Design review of the part built by this model. Coordinates are the model's own, in mm. Face numbers are marked on the shaded views. A direction names the side the tool comes from. Round coordinates to 2 decimals unless told otherwise and drop trailing zeros. Loops run counter-clockwise (first coordinate to the right, second up) from the corner with the lowest first, then second, coordinate; pieces in that order, holes last. Notation, with made-up numbers: M 42,44.5 L 79,44.5 A5 ccw 79,50.5 Z; hole C 49.5,46 d3. An arc over 180 degrees is marked long. Use a Markdown table: item, result.
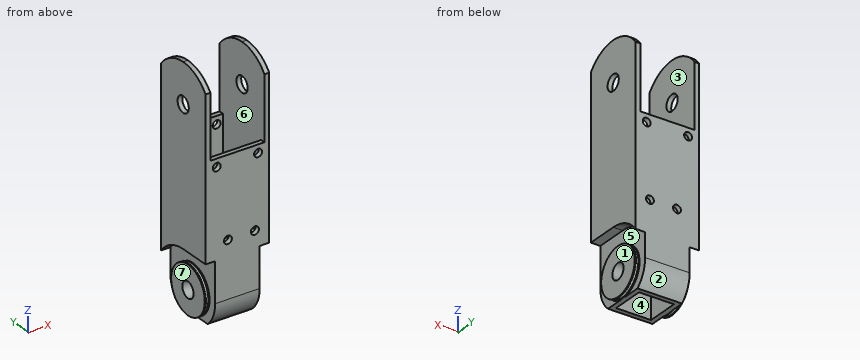
from build123d import *

# Parameters (mm, degrees)
CROQUIS1_W              = 40
CROQUIS1_H              = 40
SALIENTE_EXTRUIR1_DEPTH = 150
CROQUIS2_W              = 34
CROQUIS2_H              = 40
CORTAR_EXTRUIR1_DEPTH   = 50
CORTAR_EXTRUIR5_DEPTH   = 157.524758425
CROQUIS4_R              = 5
CORTAR_EXTRUIR6_DEPTH   = 157.524758425
CORTAR_EXTRUIR10_DEPTH  = 157.524758425
CROQUIS5_R              = 5
CORTAR_EXTRUIR7_DEPTH   = 157.524758425
CROQUIS6_R              = 5
CORTAR_EXTRUIR8_DEPTH   = 6
CORTAR_EXTRUIR11_START  = -6
CROQUIS9_R              = 5
CORTAR_EXTRUIR11_DEPTH  = 6
SALIENTE_EXTRUIR2_START = 3
CROQUIS10_R             = 15
CROQUIS10_R_2           = 5
SALIENTE_EXTRUIR2_DEPTH = 3
CROQUIS11_R             = 15
CROQUIS11_R_2           = 5
SALIENTE_EXTRUIR3_DEPTH = 3
CROQUIS12_R             = 0.75
CORTAR_EXTRUIR12_DEPTH  = 6
CORTAR_EXTRUIR13_START  = -6
CORTAR_EXTRUIR13_DEPTH  = 6
CROQUIS15_W             = 22
CROQUIS15_H             = 20.45751311
CORTAR_EXTRUIR14_DEPTH  = 153.643375225
CROQUIS16_W             = 34
CROQUIS16_H             = 34
CORTAR_EXTRUIR15_DEPTH  = 55
CROQUIS17_R             = 2.5
CORTAR_EXTRUIR16_DEPTH  = 157.524758425
CROQUIS18_R             = 2.5
CORTAR_EXTRUIR17_DEPTH  = 157.524758425


with BuildPart() as part:
    # Croquis1 → Saliente-Extruir1 (new body)
    with BuildSketch(Plane.XY):
        Rectangle(CROQUIS1_W, CROQUIS1_H)
    extrude(amount=SALIENTE_EXTRUIR1_DEPTH)

    # Croquis2 → Cortar-Extruir1 (cut)
    with BuildSketch(Plane.XY.offset(150)):
        Rectangle(CROQUIS2_W, CROQUIS2_H)
    extrude(amount=-CORTAR_EXTRUIR1_DEPTH, mode=Mode.SUBTRACT)

    # Croquis3 → Cortar-Extruir5 (cut, through all)
    with BuildSketch(Plane(origin=(20, 0, 0), x_dir=(0, 0, -1), z_dir=(1, 0, 0))):
        with BuildLine():
            ThreePointArc((-140, -20), (-147.360679775, -11.180339887), (-150, 0))
            Line((-150, 0), (-150, -20))
            Line((-150, -20), (-140, -20))
        make_face()
        with BuildLine():
            Line((-140, 20), (-150, 20))
            Line((-150, 20), (-150, 0))
            ThreePointArc((-150, 0), (-147.360679775, 11.180339887), (-140, 20))
        make_face()
    extrude(amount=-CORTAR_EXTRUIR5_DEPTH, mode=Mode.SUBTRACT)

    # Croquis4 → Cortar-Extruir6 (cut, through all)
    with BuildSketch(Plane(origin=(20, 0, 0), x_dir=(0, 0, -1), z_dir=(1, 0, 0))):
        with Locations((-125, 0)):
            Circle(CROQUIS4_R)
    extrude(amount=-CORTAR_EXTRUIR6_DEPTH, mode=Mode.SUBTRACT)

    # Croquis8 → Cortar-Extruir10 (cut, through all)
    with BuildSketch(Plane(origin=(20, 0, 0), x_dir=(0, 0, -1), z_dir=(1, 0, 0))):
        with BuildLine():
            Line((0, 20), (-15, 20))
            ThreePointArc((-15, 20), (-6.771243445, 18.228756555), (0, 13.228756555))
            Line((0, 13.228756555), (0, 20))
        make_face()
        with BuildLine():
            Line((0, -20), (0, -13.228756555))
            ThreePointArc((0, -13.228756555), (-6.771243445, -18.228756555), (-15, -20))
            Line((-15, -20), (0, -20))
        make_face()
    extrude(amount=-CORTAR_EXTRUIR10_DEPTH, mode=Mode.SUBTRACT)

    # Croquis5 → Cortar-Extruir7 (cut, through all)
    with BuildSketch(Plane(origin=(20, 0, 0), x_dir=(0, 0, -1), z_dir=(1, 0, 0))):
        with Locations((-15, 0)):
            Circle(CROQUIS5_R)
    extrude(amount=-CORTAR_EXTRUIR7_DEPTH, mode=Mode.SUBTRACT)

    # Croquis6 → Cortar-Extruir8 (cut)
    with BuildSketch(Plane(origin=(20, 0, 0), x_dir=(0, 0, -1), z_dir=(1, 0, 0))):
        with BuildLine():
            ThreePointArc((-30, 20), (-40, 0), (-30, -20))
            Line((-30, -20), (-15, -20))
            ThreePointArc((-15, -20), (-6.771243445, -18.228756555), (0, -13.228756555))
            Line((0, -13.228756555), (0, 13.228756555))
            ThreePointArc((0, 13.228756555), (-6.771243445, 18.228756555), (-15, 20))
            Line((-15, 20), (-30, 20))
        make_face()
        with Locations((-15, 0)):
            Circle(CROQUIS6_R, mode=Mode.SUBTRACT)
    extrude(amount=-CORTAR_EXTRUIR8_DEPTH, mode=Mode.SUBTRACT)

    # Croquis9 → Cortar-Extruir11 (cut)
    with BuildSketch(Plane.ZY.offset(20).offset(CORTAR_EXTRUIR11_START)):
        with BuildLine():
            ThreePointArc((30, -20), (40, 0), (30, 20))
            Line((30, 20), (15, 20))
            ThreePointArc((15, 20), (6.771243445, 18.228756555), (0, 13.228756555))
            Line((0, 13.228756555), (0, -13.228756555))
            ThreePointArc((0, -13.228756555), (6.771243445, -18.228756555), (15, -20))
            Line((15, -20), (30, -20))
        make_face()
        with Locations(Location((15, 0, 0), (0, 0, 180))):
            Circle(CROQUIS9_R, mode=Mode.SUBTRACT)
    extrude(amount=CORTAR_EXTRUIR11_DEPTH, mode=Mode.SUBTRACT)

    # Croquis10 → Saliente-Extruir2 (add)
    with BuildSketch(Plane(origin=(14, 0, 0), x_dir=(0, 0, -1), z_dir=(1, 0, 0)).offset(SALIENTE_EXTRUIR2_START)):
        with Locations((-15, 0)):
            Circle(CROQUIS10_R)
        with Locations((-15, 0)):
            Circle(CROQUIS10_R_2, mode=Mode.SUBTRACT)
    extrude(amount=-SALIENTE_EXTRUIR2_DEPTH)

    # Croquis11 → Saliente-Extruir3 (add)
    with BuildSketch(Plane.ZY.offset(14)):
        with Locations(Location((15, 0, 0), (0, 0, 180))):
            Circle(CROQUIS11_R)
        with Locations(Location((15, 0, 0), (0, 0, 180))):
            Circle(CROQUIS11_R_2, mode=Mode.SUBTRACT)
    extrude(amount=SALIENTE_EXTRUIR3_DEPTH)

    # Croquis12 → Cortar-Revolución1 (revolve, cut)
    with BuildSketch(Plane.XY.offset(15), mode=Mode.PRIVATE) as cortar_revoluci_n1_sk:
        with Locations((15.5, 15)):
            Circle(CROQUIS12_R)
        with Locations((-15.5, 15)):
            Circle(CROQUIS12_R)
    revolve(cortar_revoluci_n1_sk.sketch.rotate(Axis((-18, 0, 15), (1, 0, 0)), 270), axis=Axis((-18, 0, 15), (1, 0, 0)), mode=Mode.SUBTRACT)

    # Croquis13 → Cortar-Extruir12 (cut)
    with BuildSketch(Plane(origin=(20, 0, 0), x_dir=(0, 0, -1), z_dir=(1, 0, 0))):
        with BuildLine():
            Line((-40, 0), (-40, -20))
            Line((-40, -20), (-30, -20))
            ThreePointArc((-30, -20), (-37.360679775, -11.180339887), (-40, 0))
        make_face()
    extrude(amount=-CORTAR_EXTRUIR12_DEPTH, mode=Mode.SUBTRACT)

    # Croquis14 → Cortar-Extruir13 (cut)
    with BuildSketch(Plane.ZY.offset(20).offset(CORTAR_EXTRUIR13_START)):
        with BuildLine():
            Line((30, -20), (40, -20))
            Line((40, -20), (40, 0))
            ThreePointArc((40, 0), (37.360679775, -11.180339887), (30, -20))
        make_face()
    extrude(amount=CORTAR_EXTRUIR13_DEPTH, mode=Mode.SUBTRACT)

    # Croquis15 → Cortar-Extruir14 (cut, through all)
    with BuildSketch(Plane(origin=(0, 0, 0), x_dir=(-1, 0, 0), z_dir=(0, 0, -1))):
        Rectangle(CROQUIS15_W, CROQUIS15_H)
    extrude(amount=-CORTAR_EXTRUIR14_DEPTH, mode=Mode.SUBTRACT)

    # Croquis16 → Cortar-Extruir15 (cut)
    with BuildSketch(Plane.XY.offset(100)):
        Rectangle(CROQUIS16_W, CROQUIS16_H)
    extrude(amount=-CORTAR_EXTRUIR15_DEPTH, mode=Mode.SUBTRACT)

    # Croquis17 → Cortar-Extruir16 (cut, through all)
    with BuildSketch(Plane(origin=(0, 20, 0), x_dir=(1, 0, 0), z_dir=(0, 1, 0))):
        with Locations(Location((-13, -95, 0), (0, 0, 270))):
            Circle(CROQUIS17_R)
        with Locations(Location((13, -95, 0), (0, 0, 270))):
            Circle(CROQUIS17_R)
    extrude(amount=-CORTAR_EXTRUIR16_DEPTH, mode=Mode.SUBTRACT)

    # Croquis18 → Cortar-Extruir17 (cut, through all)
    with BuildSketch(Plane(origin=(0, 20, 0), x_dir=(1, 0, 0), z_dir=(0, 1, 0))):
        with Locations(Location((11, -50, 0), (0, 0, 270))):
            Circle(CROQUIS18_R)
        with Locations(Location((-6, -50, 0), (0, 0, 270))):
            Circle(CROQUIS18_R)
    extrude(amount=-CORTAR_EXTRUIR17_DEPTH, mode=Mode.SUBTRACT)


solid = part.part
1. Take a section at C-C on z = 66. Give the boundary of the cut face in (x, y), and give its area (3 significant figures).
Check values:
| item | result |
|---|---|
| outline | M -20,-20 L 20,-20 L 20,20 L -20,20 Z; hole M -17,-17 L 17,-17 L 17,17 L -17,17 Z |
| area | 444 mm² |
2. Take a section at B-B on x = 3. Give the boundary of the cut face in (y, z), and give its area (3 significant figures).
Check values:
| item | result |
|---|---|
| outline | M -20,15 A20 ccw -13.23,0 L -10.23,0 L -10.23,45 L -17,45 L -17,100 L -20,100 Z; M 10.23,0 L 13.23,0 A20 ccw 20,15 L 20,100 L 17,100 L 17,45 L 10.23,45 Z |
| area | 1,150 mm² |
3. Insertion check: pin 1 (2.5 mm diameter, centred on x = 3.5, y = 19, fed in from +Z); pin 2 (24 mm diameter, centred on y = 4.5, z = 20, fed in from +X); pin 3 (24 mm diameter, centred on y = 2, z = 9, fed in from -X). Each pin has a flat end and moves straight along its axis. Give the tip position at first contact, or say it passes through.
Check values:
| item | result |
|---|---|
| pin 1 | stops at z = 100 |
| pin 2 | stops at x = 17 |
| pin 3 | stops at x = -17 |
4. The part is to be moulded in two halves that separate along X. For the marked faces 5, 6 and 7, say which applies: pulls with the +X half, pulls with the -X half, needs draft (parallel to the pull), parting line crosses it, or undercut.
Check values:
| item | result |
|---|---|
| face 5 | pulls with the +X half |
| face 6 | undercut |
| face 7 | pulls with the -X half |
5. Wall thickness on line 1 along X through (y, z) = (17.8, 50); line 2 along X through (y, z) = (18, 95); line 3 along X through (y, z) = (-9, 54.5): over which ranges is each line inside the solid? List them lowest first. Write a range as from..to.
Check values:
| item | result |
|---|---|
| line 1 | x = -20..-8.5, -3.5..8.5, 13.5..20 |
| line 2 | x = -20..-15.5, -10.5..10.5, 15.5..20 |
| line 3 | x = -20..-17, 17..20 |
6. Take a section at A-A on z = 95. Give the boundary of the cut face in (x, y).
Check values:
| item | result |
|---|---|
| outline | M -20,-20 L -15.5,-20 L -15.5,-17 L -17,-17 L -17,17 L -15.5,17 L -15.5,20 L -20,20 Z; M -10.5,-20 L 10.5,-20 L 10.5,-17 L -10.5,-17 Z; M -10.5,17 L 10.5,17 L 10.5,20 L -10.5,20 Z; M 15.5,-20 L 20,-20 L 20,20 L 15.5,20 L 15.5,17 L 17,17 L 17,-17 L 15.5,-17 Z |
7. Take a section at D-D on y = 2. Count the separate pieces of the cut face and the enclosed holes in it, and give its area (3 significant figures).
Check values:
| item | result |
|---|---|
| separate pieces | 6 |
| enclosed holes | 0 |
| area | 970 mm² |
8. Machinability: for the marked faces 1, 2, 3 and 4, which of the approach directions +Z, -Z, +X, -X, +Y, -Y give a long, thin tool a straight path to every point of the face, cutting with its end or side? Answer none if there is none.
Check values:
| item | result |
|---|---|
| face 1 | -Z, +X, +Y, -Y |
| face 2 | -Z, +X, -X, +Y |
| face 3 | +Z |
| face 4 | +Z, -Z |
